```python
from build123d import *

# Parameters (mm, degrees)
F0_R     = 7
F0_W     = 8
F0_H     = 10
F1_DEPTH = 5


with BuildPart() as f1:
    # F0 (on Front) → F1 (new body)
    with BuildSketch(Plane.XZ):
        with BuildLine():
            ThreePointArc((-34, 0), (0, 34), (34, 0))
            Line((34, 0), (50, 0))
            Line((50, 0), (50, -20))
            ThreePointArc((50, -20), (68.737322, -57.801565), (110.166667, -65.779969))
            ThreePointArc((110.166667, -65.779969), (115.458224, -62.197381), (117.5, -56.142081))
            Line((117.5, -56.142081), (117.5, -9.010085))
            ThreePointArc((117.5, -9.010085), (115.734988, -0.795146), (110.751478, 5.969847))
            Line((110.751478, 5.969847), (74.969897, 37.622784))
            Line((74.969897, 37.622784), (71.657027, 33.877801))
            Line((71.657027, 33.877801), (60.422079, 43.816409))
            Line((60.422079, 43.816409), (63.734948, 47.561392))
            Line((63.734948, 47.561392), (53.918715, 56.244983))
            ThreePointArc((53.918715, 56.244983), (52.377157, 57.175731), (50.605846, 57.5))
            Line((50.605846, 57.5), (42.5, 57.5))
            Line((42.5, 57.5), (42.5, 52.5))
            Line((42.5, 52.5), (-42.5, 52.5))
            Line((-42.5, 52.5), (-42.5, 57.5))
            Line((-42.5, 57.5), (-50.428932, 57.5))
            ThreePointArc((-50.428932, 57.5), (-52.342349, 57.880602), (-53.964466, 58.964466))
            Line((-53.964466, 58.964466), (-54.571068, 59.571068))
            ThreePointArc((-54.571068, 59.571068), (-57.815301, 61.738795), (-61.642136, 62.5))
            Line((-61.642136, 62.5), (-109, 62.5))
            ThreePointArc((-109, 62.5), (-110.414214, 61.914214), (-111, 60.5))
            Line((-111, 60.5), (-111, 50))
            Line((-111, 50), (-103, 50))
            Line((-103, 50), (-103, 40))
            Line((-103, 40), (-111, 40))
            Line((-111, 40), (-111, 5))
            ThreePointArc((-111, 5), (-112.464466, 1.464466), (-116, 0))
            Line((-116, 0), (-117.5, 0))
            ThreePointArc((-117.5, 0), (-118.56066, -0.43934), (-119, -1.5))
            Line((-119, -1.5), (-119, -59.166312))
            ThreePointArc((-119, -59.166312), (-118.165686, -61.931644), (-115.941176, -63.774113))
            ThreePointArc((-115.941176, -63.774113), (-71.22935, -59.574019), (-50, -20))
            Line((-50, -20), (-50, 0))
            Line((-50, 0), (-34, 0))
        make_face()
        with Locations((-97.5, -20)):
            Circle(F0_R, mode=Mode.SUBTRACT)
        with Locations((97.5, -20)):
            Circle(F0_R, mode=Mode.SUBTRACT)
        with Locations((-79, 45)):
            Rectangle(F0_W, F0_H, mode=Mode.SUBTRACT)
    extrude(amount=F1_DEPTH)


solid = f1.part
```
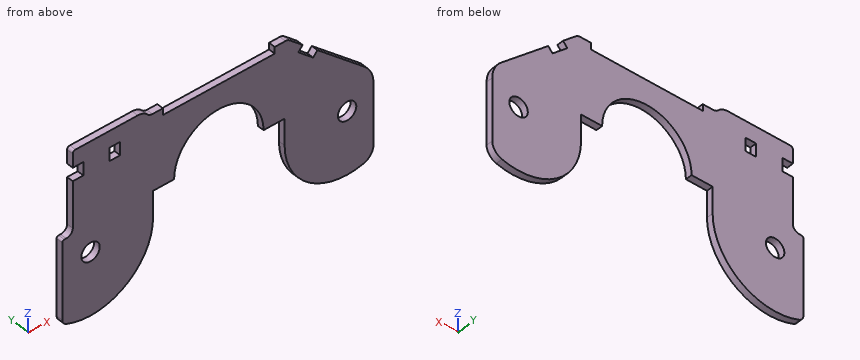
The model under review builds one solid part; all positions refer to its coordinate system, in mm. Round coordinates to 2 decimals unless told otherwise and drop trailing zeros. Order: outer loops, then holes, each group sorted by start corner. A loop starts at its lowest first (then second) coordinate and runs counter-clockwise, first axis right, second up. Notation, with made-up numbers: (20, 58.25) -> (40, 58.25) arc R19 cw to (40, 75.25) -> close; hole circle Ø2 at (56, 64.25). An arc over 180 degrees is marked (long way). Use a Markdown table: item, result.
Q1. For line 1 (Z direction, x = -97.5, y = -2.7); line 2 (Z direction, x = 97.5, y = -2.85); line 3 (X direction, y = -3.9, z = -7), list the stretches that pass through material, from the lowest coordinate up.
Values:
| item | result |
|---|---|
| line 1 | z = -67.5 to -27, -13 to 62.5 |
| line 2 | z = -67.5 to -27, -13 to 17.69 |
| line 3 | x = -119 to -50, 50 to 117.4 |
Q2. We need section B-B on z = -34. Write out the cut boundary in (x, y).
Values:
| item | result |
|---|---|
| outline | (-119, -5) -> (-52.11, -5) -> (-52.11, 0) -> (-119, 0) -> close; (52.11, -5) -> (117.5, -5) -> (117.5, 0) -> (52.11, 0) -> close |
Q3. We need section D-D on x = 0. Write out the cut boundary in (y, z), then the cut area to 3 significant figures.
Values:
| item | result |
|---|---|
| outline | (-5, 34) -> (0, 34) -> (0, 52.5) -> (-5, 52.5) -> close |
| area | 92.5 mm^2 |
Q4. Clearance check with flat-ended pins moving along their axes: P1, Ø1.5, axis at y = -3.5, z = 43, coming from the -X side; P2, Ø3, axis at x = 53, y = -1.5, coming from the +Z side; P3, Ø1.2, axis at x = -117, y = -3.5, coming from the +Z side. State where each tip first meets the part, or that it passes through.
Values:
| item | result |
|---|---|
| P1 | stops at x = -103 |
| P2 | stops at z = 57.42 |
| P3 | stops at z = 0 |
Q5. We need section C-C on y = -2.3. State how many separate pieces and enclosed holes the cut face has, then the cut area to 3 significant figures.
Values:
| item | result |
|---|---|
| separate pieces | 1 |
| enclosed holes | 3 |
| area | 16,900 mm^2 |
Q6. We need section A-A on x = -97.5. Write out the cut boundary in (y, z), then the cut area to 3 significant figures.
Values:
| item | result |
|---|---|
| outline | (-5, -67.5) -> (0, -67.5) -> (0, -27) -> (-5, -27) -> close; (-5, -13) -> (0, -13) -> (0, 62.5) -> (-5, 62.5) -> close |
| area | 580 mm^2 |
